Verification items for the finished model (mm, model axes). A direction names the side the tool comes from. Give positions to 0.01 mm unless a question says otherwise; leave off trailing zeros. Write each loop counter-clockwise with the first axis right and the second up, starting at its lowest first coordinate (ties: lowest second). Pieces come first, ordered by that corner, then holes.
from build123d import *
from OCP.BRepFilletAPI import BRepFilletAPI_MakeChamfer

# Parameters (mm, degrees)
SKETCH1_W           = 30
SKETCH1_H           = 30
BOSS_EXTRUDE1_DEPTH = 30
SKETCH2_W           = 20
SKETCH2_H           = 20
CUT_EXTRUDE1_DEPTH  = 37.742346142
SKETCH3_W           = 30
SKETCH3_H           = 5
BOSS_EXTRUDE2_DEPTH = 40
SKETCH4_R           = 5.5
SKETCH4_R_2         = 1.8
CUT_EXTRUDE2_DEPTH  = 65.420493634
CUT_EXTRUDE3_DEPTH  = 63.24949799
SKETCH5_W           = 5
SKETCH5_H           = 25
BOSS_EXTRUDE4_DEPTH = 34
CHAMFER1_SIZE       = 25
SKETCH8_R           = 2.1
CUT_EXTRUDE4_DEPTH  = 63.657800791
SKETCH9_W           = 5
SKETCH9_H           = 30
BOSS_EXTRUDE5_DEPTH = 12
CHAMFER2_SIZE       = 10
CHAMFER2_SIZE2      = 5.773502692
SKETCH10_R          = 2.1
CUT_EXTRUDE5_DEPTH  = 63.657800791
SKETCH11_W          = 25
SKETCH11_H          = 5
BOSS_EXTRUDE6_DEPTH = 16
CHAMFER3_SIZE       = 4
SKETCH12_R          = 1.8
CUT_EXTRUDE6_DEPTH  = 58.017541161
CUT_EXTRUDE7_DEPTH  = 3
CUT_EXTRUDE8_DEPTH  = 60.380131357
CHAMFER4_SIZE       = 1
CHAMFER4_SIZE2      = 0.711458249


with BuildPart() as part:
    # Sketch1 → Boss-Extrude1 (new body)
    with BuildSketch(Plane(origin=(0, 0, 0), x_dir=(1, 0, 0), z_dir=(0, 1, 0))):
        Rectangle(SKETCH1_W, SKETCH1_H)
    extrude(amount=BOSS_EXTRUDE1_DEPTH)

    # Sketch2 → Cut-Extrude1 (cut, through all)
    with BuildSketch(Plane(origin=(0, 30, 0), x_dir=(1, 0, 0), z_dir=(0, 1, 0))):
        Rectangle(SKETCH2_W, SKETCH2_H)
    extrude(amount=-CUT_EXTRUDE1_DEPTH, mode=Mode.SUBTRACT)

    # Sketch3 → Boss-Extrude2 (add)
    with BuildSketch(Plane(origin=(15, 0, 0), x_dir=(0, 0, -1), z_dir=(1, 0, 0))):
        with Locations((0, 2.5)):
            Rectangle(SKETCH3_W, SKETCH3_H)
    extrude(amount=BOSS_EXTRUDE2_DEPTH)

    # Sketch4 → Cut-Extrude2 (cut, through all)
    with BuildSketch(Plane.XZ):
        with Locations(Location((31, 0, 0), (0, 0, 270))):
            Circle(SKETCH4_R)
        with Locations(Location((19, 0, 0), (0, 0, 270))):
            Circle(SKETCH4_R_2)
        with Locations(Location((43, 0, 0), (0, 0, 270))):
            Circle(SKETCH4_R_2)
    extrude(amount=-CUT_EXTRUDE2_DEPTH, mode=Mode.SUBTRACT)

    # Sketch7 → Cut-Extrude3 (cut, through all)
    with BuildSketch(Plane(origin=(0, 5, 0), x_dir=(1, 0, 0), z_dir=(0, 1, 0))):
        Polygon((15, -15), (49, -6), (49, 15), (55, 15), (55, -15), align=None)
    extrude(amount=-CUT_EXTRUDE3_DEPTH, mode=Mode.SUBTRACT)

    # Sketch5 → Boss-Extrude4 (add)
    with BuildSketch(Plane(origin=(15, 0, 0), x_dir=(0, 0, -1), z_dir=(1, 0, 0))):
        with Locations((12.5, 17.5)):
            Rectangle(SKETCH5_W, SKETCH5_H)
    extrude(amount=BOSS_EXTRUDE4_DEPTH)

    # Chamfer1
    chamfer1_edges = [part.edges().sort_by_distance(p)[0] for p in [
        (49, 30, -12.5),
    ]]
    chamfer(chamfer1_edges, length=CHAMFER1_SIZE)

    # Sketch8 → Cut-Extrude4 (cut, through all)
    with BuildSketch(Plane.XY.offset(-10)):
        with Locations((23, 17)):
            Circle(SKETCH8_R)
    extrude(amount=-CUT_EXTRUDE4_DEPTH, mode=Mode.SUBTRACT)

    # Sketch9 → Boss-Extrude5 (add)
    with BuildSketch(Plane.ZY.offset(15)):
        with Locations((-12.5, 15)):
            Rectangle(SKETCH9_W, SKETCH9_H)
    extrude(amount=BOSS_EXTRUDE5_DEPTH)

    # Chamfer2
    chamfer2_edges = [part.edges().sort_by_distance(p)[0] for p in [
        (-27, 30, -12.5),
    ]]
    chamfer2_side = [part.faces().sort_by_distance(p)[0] for p in [
        (-27, 15, -12.5),
    ]]
    chamfer(chamfer2_edges, length=CHAMFER2_SIZE, length2=CHAMFER2_SIZE2, reference=chamfer2_side[0])

    # Sketch10 → Cut-Extrude5 (cut, through all)
    with BuildSketch(Plane.XY.offset(-10)):
        with Locations((-21, 17)):
            Circle(SKETCH10_R)
    extrude(amount=-CUT_EXTRUDE5_DEPTH, mode=Mode.SUBTRACT)

    # Sketch11 → Boss-Extrude6 (add)
    with BuildSketch(Plane.ZY.offset(15)):
        with Locations((2.5, 2.5)):
            Rectangle(SKETCH11_W, SKETCH11_H)
    extrude(amount=BOSS_EXTRUDE6_DEPTH)

    # Chamfer3
    chamfer3_edges = [part.edges().sort_by_distance(p)[0] for p in [
        (-31, 2.5, 15),
        (-31, 2.5, -10),
    ]]
    chamfer(chamfer3_edges, length=CHAMFER3_SIZE - 0.0001)  # a hair under: the kernel refuses the full size

    # Sketch12 → Cut-Extrude6 (cut, through all)
    with BuildSketch(Plane(origin=(0, 5, 0), x_dir=(1, 0, 0), z_dir=(0, 1, 0))):
        with Locations(Location((-25, 0, 0), (0, 0, 270))):
            Circle(SKETCH12_R)
    extrude(amount=-CUT_EXTRUDE6_DEPTH, mode=Mode.SUBTRACT)

    # Sketch13 → Cut-Extrude7 (cut)
    with BuildSketch(Plane(origin=(0, 5, 0), x_dir=(1, 0, 0), z_dir=(0, 1, 0))):
        Polygon((-25, -3.464101615), (-22, -1.732050808), (-22, 1.732050808), (-25, 3.464101615), (-28, 1.732050808), (-28, -1.732050808), align=None)
    extrude(amount=-CUT_EXTRUDE7_DEPTH, mode=Mode.SUBTRACT)

    # Sketch14 → Cut-Extrude8 (cut, through all)
    with BuildSketch(Plane(origin=(0, 30, 0), x_dir=(1, 0, 0), z_dir=(0, 1, 0))):
        Polygon((-6, -10), (-10, -15), (10, -15), (6, -10), align=None)
    extrude(amount=-CUT_EXTRUDE8_DEPTH, mode=Mode.SUBTRACT)

    # Chamfer4: one chamfer whose edges measure the first distance from different faces: ONE call of the kernel's chamfer builder (chamfer() names one face for all edges)
    chamfer4_edges_1 = [part.edges().sort_by_distance(p)[0] for p in [
        (-6, 15, 10),
    ]]
    chamfer4_side_1 = [part.faces().sort_by_distance(p)[0] for p in [
        (-8, 15, 12.5),
    ]]
    chamfer4_edges_2 = [part.edges().sort_by_distance(p)[0] for p in [
        (6, 15, 10),
    ]]
    chamfer4_side_2 = [part.faces().sort_by_distance(p)[0] for p in [
        (8, 15, 12.5),
    ]]
    chamfer4 = BRepFilletAPI_MakeChamfer(part.part.solid().wrapped)
    for e in chamfer4_edges_1:
        chamfer4.Add(CHAMFER4_SIZE, CHAMFER4_SIZE2, e.wrapped, chamfer4_side_1[0].wrapped)  # the first distance lies on this face
    for e in chamfer4_edges_2:
        chamfer4.Add(CHAMFER4_SIZE, CHAMFER4_SIZE2, e.wrapped, chamfer4_side_2[0].wrapped)  # the first distance lies on this face
    add(Compound.cast(chamfer4.Shape()), mode=Mode.REPLACE)


solid = part.part
Item 1: Sectioned sample at A-A on z = 0. State how many separate pieces and enclosed holes the cut face has, then the cut area to 3 significant figures.
Answer key:
separate pieces: 6
enclosed holes: 0
area: 434 mm2
Item 2: Release check for a two-part mould opening along X. For faces 1 (the face through (12, 15, -15)), 2 (the face through (8.336, 15.21, 12.92)), 3 (the face through (-29, 2, 13)) record: released by +X, released by -X, zero draft, split by the parting line, or undercut.
Answer key:
face 1: zero draft
face 2: undercut
face 3: released by -X
Item 3: Set-up check for faces 4 (the face through (28, 15, -10)), 5 (the face through (-8, 15, 10)), 6 (the face through (-22, 4, 0)), 7 (the face through (-8.29, 15.21, 12.86)): record each of +Z, -Z, +X, -X, +Y, -Y from which the full face is reachable in a straight line by a thin tool's end or side.
Answer key:
face 4: +Z, +X, +Y
face 5: +Y, -Y
face 6: +Y
face 7: +Z, +Y, -Y
Item 4: Sectioned sample at B-B on y = 17. Record the cut outline in (x, z), then the cut area to 3 significant figures.
Answer key:
outline: (-27, -15) - (-23.1, -15) - (-23.1, -10) - (-27, -10) - close; (-18.9, -15) - (20.9, -15) - (20.9, -10) - (15, -10) - (15, 15) - (10, 15) - (6.62, 10.78) - (6.71, 10) - (10, 10) - (10, -10) - (-10, -10) - (-10, 10) - (-6.71, 10) - (-6.62, 10.78) - (-10, 15) - (-15, 15) - (-15, -10) - (-18.9, -10) - close; (25.1, -15) - (37, -15) - (37, -10) - (25.1, -10) - close
area: 547 mm2
Item 5: Depth check by flat-ended pin: pin 1 (8 mm diameter, centred on x = -23, z = -1.5, fed in from +Y); pin 2 (3 mm diameter, centred on y = 26.5, z = -2.5, fed in from +X); pin 3 (5.5 mm diameter, centred on y = 9.5, z = -12, fed in from -X). Enter the tip coordinate at first touch or a pass-through.
Answer key:
pin 1: stops at y = 5
pin 2: stops at x = 15
pin 3: stops at x = -27
Item 6: Sectioned sample at D-D on z = 9.25. Record the cut outline in (x, y), then the cut area to 3 significant figures.
Answer key:
outline: (-31, 0) - (-10, 0) - (-10, 30) - (-15, 30) - (-15, 5) - (-31, 5) - close; (10, 0) - (36.72, 0) - (36.72, 5) - (15, 5) - (15, 30) - (10, 30) - close
area: 489 mm2
Item 7: Sectioned sample at C-C on x = 31. Record the cut outline in (y, z).
Answer key:
outline: (0, -15) - (23, -15) - (23, -10) - (5, -10) - (5, -5.5) - (0, -5.5) - close; (0, 5.5) - (5, 5.5) - (5, 10.76) - (0, 10.76) - close
Item 8: Scan lines: line 1 along X through (y, z) = (0.5, 0); line 2 along X through (y, z) = (7, 3.75); line 3 along Z through (x, y) = (-19, 15). Record each from-to range of solid material in increasing order.
Answer key:
line 1: x = -31 to -26.8, -23.2 to -10, 10 to 17.2, 20.8 to 25.5, 36.5 to 41.2, 44.8 to 49
line 2: x = -15 to -10, 10 to 15
line 3: z = -15 to -10
